```python
from build123d import *

# Parameters (mm, degrees)
F1_DEPTH = 25
F2_DEPTH = 25
F4_DEPTH = 25


# Not quite as in the source:
# - a feature of the source that left no trace in its solid (it failed there, or was rolled back) is left out


with BuildPart() as f1:
    # F0 (on Right) → F1 (new body)
    with BuildSketch(Plane.YZ):
        Polygon((-25, 0), (0, 0), (0, 50), align=None)
        Polygon((0, 50), (0, 0), (25, 0), align=None)
    extrude(amount=F1_DEPTH)

    # F2 (add): a face of the model
    f2_faces = [f1.faces().sort_by_distance(p)[0] for p in [
        (0, 0, 16.6666666667),
    ]]
    extrude(f2_faces, amount=F2_DEPTH)

    # F3 (on face) → F4 (cut)
    with BuildSketch(Plane(origin=(-25, 0, 0), x_dir=(0, -1, 0), z_dir=(-1, 0, 0))):
        Polygon((-13.9194109071, 5.4563577287), (0, 5.4563577287), (0, 42.9563577287), align=None)
        Polygon((0, 42.9563577287), (0, 5.4563577287), (13.9194109071, 5.4563577287), align=None)
    extrude(amount=-F4_DEPTH, mode=Mode.SUBTRACT)


solid = f1.part
```
The listing builds one solid part. Answer for the finished solid, in the listing's coordinates (mm). A direction names the side the tool comes from. Give positions to 0.01 mm unless a question says otherwise; leave off trailing zeros. Order: outer loops, then holes, each group sorted by start corner. A loop starts at its lowest first (then second) coordinate and runs counter-clockwise, first axis right, second up. Notation, with made-up numbers: (84.5, -15) -> (95.5, -15) arc R19 ccw to (95.5, 5) -> close; hole circle Ø2 at (-4.5, -21.75). An arc over 180 degrees is marked (long way). Answer as CSV lines item,"result". Start each with the question number.
Q1. A cutting plane is placed at D-D (x = 15.5). Determine the outline of the cut face in (y, z).
Q2. Find the intervals of material crossed by L1, parallel to Y at x = -21.5, z = 17; L2, parallel to Y at x = -3, z = 25; L3, parallel to X at y = -7.5, z = 5.5, in increasing order.
Q3. A cutting plane is placed at B-B (z = 19). Determine the outline of the cut face in (x, y).
Q4. A cutting plane is placed at C-C (y = -4.5). Determine the outline of the cut face in (x, z), then the cut area to 3 significant figures.
Q5. Determine the mould class of faces 1 (the flat face through (-13, 0, 5.456)), 2 (the flat face through (0.35, -12.325, 25.35)), 3 (the flat face through (25, 0, 20)) for opening direction Z: pulls with the +Z half, pulls with the -Z half, needs draft (parallel to the pull), parting line crosses it, or undercut.
Q6. Given pin 1 (4 mm diameter, centred on x = 6, y = -14, fed in from +Z); pin 2 (1.5 mm diameter, centred on x = 11.5, z = 41.5, fed in from -Y) (3 decimals); pin 3 (10 mm diameter, centred on x = 20, z = 32, fed in from +Y), each flat-ended and moving along its own axis, determine where each tip first touches the part or whether it passes through.
Q7. A cutting plane is placed at A-A (x = -2.5). Determine the outline of the cut face in (y, z).
Q8. Which of the six approach directions +Z, -Z, +X, -X, +Y, -Y give full straight-line access (tool end or side, diameter ignored) to faces 4 (the flat face through (0.35, 12.675, 24.65)), 5 (the flat face through (0, 0, 20))?
Results found:
1,outline,"(-25, 0) -> (25, 0) -> (0, 50) -> close"
2,L1,"-16.5 to -9.63, 9.63 to 16.5"
2,L2,"-12.5 to -6.67, 6.67 to 12.5"
2,L3,"0 to 25"
3,outline,"(-25, -15.5) -> (25, -15.5) -> (25, 15.5) -> (-25, 15.5) -> (-25, 8.89) -> (0, 8.89) -> (0, -8.89) -> (-25, -8.89) -> close"
4,outline,"(-25, 0) -> (25, 0) -> (25, 41) -> (-25, 41) -> (-25, 30.83) -> (0, 30.83) -> (0, 5.46) -> (-25, 5.46) -> close"
4,area,"1,420 mm2"
5,face 1,"undercut"
5,face 2,"pulls with the +Z half"
5,face 3,"needs draft"
6,pin 1,"z = 26"
6,pin 2,"y = -4.625"
6,pin 3,"y = 11.5"
7,outline,"(-25, 0) -> (25, 0) -> (0, 50) -> close; hole (-13.92, 5.46) -> (13.92, 5.46) -> (0, 42.96) -> close"
8,face 4,"+Z, +X, -X, +Y"
8,face 5,"-X"
